Design review of the part built by this model. Coordinates are the model's own, in mm. Round coordinates to 2 decimals unless told otherwise and drop trailing zeros. Order: outer loops, then holes, each group sorted by start corner. A loop starts at its lowest first (then second) coordinate and runs counter-clockwise, first axis right, second up. Notation, with made-up numbers: (40.25, 53) - (76.25, 53) arc R18 ccw to (76.25, 70) - close; hole circle Ø10 at (-22.75, 3). An arc over 180 degrees is marked (long way). Use CSV: the item, a comma, the result in double quotes.
Autodesk Inventor part; units mm, degrees
ref_plane "YZ Plane" through (0, 0, 0) normal (1, 0, 0) x (0, 1, 0)
ref_plane "XZ Plane" through (0, 0, 0) normal (0, 1, 0) x (-1, 0, 0)
ref_plane "XY Plane" through (0, 0, 0) normal (0, 0, 1) x (1, 0, 0)
sketch "Sketch1" plane through (0, 0, 0) normal (0, 1, 0) x (-1, 0, 0)
  line L0 (-7.5, -30) -> (7.5, -30)
  line L1 (7.5, -30) -> (7.5, 30)
  line L2 (7.5, 30) -> (-7.5, 30)
  line L3 (-7.5, 30) -> (-7.5, -30)
  line L4 (-7.5, -30) -> (7.5, 30) construction
  line L5 (7.5, -30) -> (-7.5, 30) construction
  point P0 (0, 0)
  dimension "d0" = 15
  dimension "d1" = 60
extrude "Extrusion1" add sketch "Sketch1" along normal blind 3
sketch "Sketch2" plane through (0, 3, 0) normal (0, 1, 0) x (1, 0, 0)
  line L0 (-7.5, 30) -> (-7.5, -30)
  line L1 (7.5, 20.5) -> (-7.5, 20.5)
  line L2 (-7.5, 20.5) -> (-7.5, -20.5)
  line L3 (-7.5, -20.5) -> (7.5, -20.5)
  line L4 (7.5, -20.5) -> (7.5, 20.5)
  line L5 (7.5, 20.5) -> (-7.5, -20.5) construction
  line L6 (-7.5, 20.5) -> (7.5, -20.5) construction
  line L7 (7.5, -20.5) -> (-7.5, -20.5)
  line L8 (-7.5, -20.5) -> (-7.5, -30)
  line L9 (-7.5, -30) -> (7.5, -30)
  line L10 (7.5, -30) -> (7.5, -20.5)
  line L11 (7.5, 30) -> (-7.5, 30)
  line L12 (7.5, 20.5) -> (-7.5, 20.5)
  line L13 (-7.5, 20.5) -> (-7.5, 30)
  line L14 (-7.5, 30) -> (7.5, 30)
  line L15 (7.5, 30) -> (7.5, 20.5)
  point P0 (0, 0)
  dimension "d4" = 41
extrude "Extrusion2" add sketch "Sketch2" along normal blind 19 contours L11 L15 L1 L0 | L3 L10 L9 L0
sketch "Sketch3" plane through (-7.5, 0, -30) normal (-1, 0, 0) x (0, 0, 1)
  line L0 (60, 0) -> (0, 0)
  line L1 (60, 0) -> (50, 0)
  line L2 (50, 0) -> (50, -21.64)
  line L3 (50, -21.64) -> (60, -21.64)
  line L4 (60, -21.64) -> (60, 0)
  point P0 (30, 0)
  dimension "d7" = 10
  dimension "d8" = 21.64
extrude "Extrusion3" add sketch "Sketch3" against normal blind 15
sketch "Sketch5" plane through (-7.5, 0, -30) normal (-1, 0, 0) x (0, 0, 1)
  line L0 (0, 0) -> (50, 0)
  line L1 (28.3595, 0) -> (50, -21.6405)
  line L2 (50, -21.64) -> (50, 0)
  line L3 (28.3595, 0) -> (58.9638, 0) construction
  line L4 (50, -21.6405) -> (50, 0)
  line L5 (50, 0) -> (28.3595, 0)
  point P0 (30, 0)
  dimension "d15" = 45
extrude "Extrusion5" add sketch "Sketch5" against normal blind 15
sketch "Sketch6" plane through (-7.5, 0, -30) normal (-1, 0, 0) x (0, 0, 1)
  line L0 (60, -21.64) -> (60, 22)
  line L1 (60, -21.64) -> (50.1294, -21.64)
  line L2 (50.1294, -21.64) -> (50.1294, -11.769)
  line L3 (50.1294, -11.769) -> (60, -11.769)
  line L4 (60, -11.769) -> (60, -21.64)
  point P0 (30, 0)
  dimension "d18" = 9.871
extrude "Extrusion6" add sketch "Sketch6" along normal blind 50
sketch "Sketch7" plane through (-7.5, 22, 30) normal (0, 0, 1) x (1, 0, 0)
  point P0 (7.5, -22)
fillet "Fillet1" radius 5 2 edges at (-57.5, -21.64, 25.0647) (-57.5, -11.769, 25.0647)
sketch "Sketch8" plane through (-7.5, -21.64, 20.1294) normal (0, 0, -1) x (-1, 0, 0)
  arc A0 (45, 0) -> (50, 5) centre (45, 5) ccw
  point P0 (-7.5, 21.64)
hole "Hole1" at (-52.5, -16.64, 20.1294) direction (0, 0, 1) diameter 3 end through all
ref_plane "Work Plane1" through (-7.5, 0, -30) normal (-1, 0, 0) x (0, 0, 1)
split "Split1" plane through (-7.5, 0, -30) removes the side toward (1, 0, 0)
properties part number "TurretServoSupport_A" material "PC/ABS Plastic"
1) To check wall thickness, follow L1, parallel to Y at x = -52.5, z = 26; L2, parallel to X at y = -16.64, z = 22.75; L3, parallel to X at y = -17.75, z = 21.5. State the ranges of each line that lie inside material, in increasing order. Write a range as from..to.
Data:
L1,"y = -21.64..-18.14, -15.14..-11.77"
L2,"x = -57.5..-54, -51..-7.5"
L3,"x = -57.38..-53.51, -51.49..-7.5"
2) We need section C-C (x = -52). Give the boundary of the cut face in (y, z), then the cut area to 3 significant figures.
Data:
outline,"(-21.64, 20.13) - (-18.05, 20.13) - (-18.05, 30) - (-21.64, 30) - close; (-15.23, 20.13) - (-11.77, 20.13) - (-11.77, 30) - (-15.23, 30) - close"
area,"69.5 mm2"
3) We need section A-A (y = -16.25). Give the boundary of the cut face in (x, z).
Data:
outline,"(-57.47, 20.13) - (-53.95, 20.13) - (-53.95, 30) - (-57.47, 30) - close; (-51.05, 20.13) - (-7.5, 20.13) - (-7.5, 30) - (-51.05, 30) - close"
4) The part is to be moulded in two halves that separate along Y. For faces 1 (the face through (-51.17, -15.95, 25.13)), 2 (the face through (-56.05, -13.25, 25)), 3 (the face through (-7.5, -17, 25)), say which applies: +Y half, -Y half, draft (parallel to the pull), parting line (faces both ways), or undercut.
Data:
face 1,"undercut"
face 2,"+Y half"
face 3,"draft"
5) We need section B-B (z = 26.75). Give the boundary of the cut face in (x, y).
Data:
outline,"(-57.5, -16.7) arc R5 ccw to (-52.5, -21.64) - (-7.5, -21.64) - (-7.5, -11.77) - (-52.5, -11.77) arc R5 ccw to start; hole circle Ø3 at (-52.5, -16.64)"
